```python
from build123d import *

# Parameters (mm, degrees)
CROQUIS1_R              = 2.5
SALIENTE_EXTRUIR1_DEPTH = 6
REDONDEO1_R             = 0.5
REDONDEO2_R             = 0.2
CROQUIS3_W              = 2.5
CROQUIS3_H              = 1
REDONDEO3_R             = 0.5


with BuildPart() as part:
    # Croquis1 → Saliente-Extruir1 (new body)
    with BuildSketch(Plane(origin=(0, 0, 0), x_dir=(1, 0, 0), z_dir=(0, 1, 0))):
        Polygon((-2.886751346, 5), (-5.773502692, 0), (-2.886751346, -5), (2.886751346, -5), (5.773502692, 0), (2.886751346, 5), align=None)
        Circle(CROQUIS1_R, mode=Mode.SUBTRACT)
    extrude(amount=SALIENTE_EXTRUIR1_DEPTH)

    # Redondeo1
    redondeo1_edges = [part.edges().sort_by_distance(p)[0] for p in [
        (2.886751346, 3, -5),
        (5.773502692, 3, 0),
        (2.886751346, 3, 5),
        (-2.886751346, 3, 5),
        (-5.773502692, 3, 0),
        (-2.886751346, 3, -5),
    ]]
    fillet(redondeo1_edges, radius=REDONDEO1_R)

    # Redondeo2
    redondeo2_edges = [part.edges().sort_by_distance(p)[0] for p in [
        (-4.330127019, 0, -2.5),
        (-4.330127019, 6, -2.5),
        (0, 0, -5),
        (4.330127019, 0, -2.5),
        (4.330127019, 0, 2.5),
        (0, 0, 5),
        (-4.330127019, 0, 2.5),
        (-2.848076211, 0, 4.933012702),
        (-5.696152423, 0, 0),
        (2.848076211, 0, 4.933012702),
        (5.696152423, 0, 0),
        (2.848076211, 0, -4.933012702),
        (-2.848076211, 0, -4.933012702),
        (0, 6, -5),
        (-4.330127019, 6, 2.5),
        (0, 6, 5),
        (4.330127019, 6, 2.5),
        (4.330127019, 6, -2.5),
        (-2.848076211, 6, 4.933012702),
        (-5.696152423, 6, 0),
        (2.848076211, 6, 4.933012702),
        (5.696152423, 6, 0),
        (2.848076211, 6, -4.933012702),
        (-2.848076211, 6, -4.933012702),
    ]]
    fillet(redondeo2_edges, radius=REDONDEO2_R)

    # Croquis3 → Cortar-Revolución1 (revolve, cut)
    with BuildSketch(Plane.XY):
        with Locations((-5.75, 5.5)):
            Rectangle(CROQUIS3_W, CROQUIS3_H)
    revolve(axis=Axis((0, 0, 0), (0, 1, 0)), mode=Mode.SUBTRACT)

    # Redondeo3
    redondeo3_edges = [part.edges().sort_by_distance(p)[0] for p in [
        (4.5, 6, 0),
    ]]
    fillet(redondeo3_edges, radius=REDONDEO3_R)


solid = part.part
```
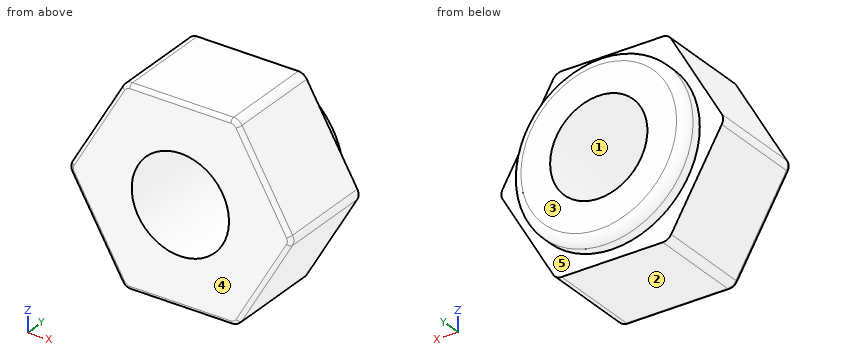
Here's how the part is built. I have some questions about the finished solid (model axes, mm). Face numbers are marked on the shaded views. A direction names the side the tool comes from. Round coordinates to 2 decimals unless told otherwise and drop trailing zeros. Order: outer loops, then holes, each group sorted by start corner. A loop starts at its lowest first (then second) coordinate and runs counter-clockwise, first axis right, second up. Notation, with made-up numbers: (68.5, 59) -> (97.5, 59) arc R8 cw to (97.5, 65) -> close; hole circle Ø10 at (20.25, -35.75). An arc over 180 degrees is marked (long way). Use a Markdown table: item, result. Add a question column.
(1) For pin 1 Ø1 at (x, y) = (-4.5, 4.5) entering from -Z; pin 2 Ø1 at (y, z) = (1, -2.5) entering from -X, each with a flat end and sliding along its axis, tell me the tip position at first contact or that it passes through.
(2) Suppose I cut it at B-B, the plane x = 0. Please give me the cut outline in (y, z), and give its area (3 significant figures).
(3) For the marked faces 4 and 5, which set-ups out of +Z, -Z, +X, -X, +Y, -Y let a thin tool reach every point of the face, with its end or its side?
(4) I need wall thicknesses on line 1 along X through (y, z) = (2.25, 0); line 2 along Z through (x, y) = (0, 4.6); line 3 along X through (y, z) = (4.05, -1). Which ranges of each line are inside material? Lowest first, please.
(5) Suppose I cut it at A-A, the plane z = 0. Please give me the cut outline in (x, y).
(6) If we mould it in two halves opening along Z, with no side actions, what happens to the marked faces 1, 2 and 3? For each: released by +Z, released by -Z, zero draft, split by the parting line, or undercut.
(7) Suppose I cut it at C-C, the plane y = 1.8. Please give me the cut outline in (x, z), and give its area (3 significant figures).
(8) Suppose I cut it at D-D, the plane y = 5.2. Please give me the cut outline in (x, z), and give its area (3 significant figures).
Verdict:
| question | item | result |
|---|---|---|
| 1 | pin 1 | z = -3.07 |
| 1 | pin 2 | x = -4.62 |
| 2 | outline | (0, -4.8) arc R0.2 ccw to (0.2, -5) -> (5, -5) -> (5, -4.5) -> (5.5, -4.5) arc R0.5 ccw to (6, -4) -> (6, -2.5) -> (0, -2.5) -> close; (0, 2.5) -> (6, 2.5) -> (6, 4) arc R0.5 ccw to (5.5, 4.5) -> (5, 4.5) -> (5, 5) -> (0.2, 5) arc R0.2 ccw to (0, 4.8) -> close |
| 2 | area | 28.9 mm2 |
| 3 | face 4 | +Z, -Z, +X, -X, -Y |
| 3 | face 5 | +Y |
| 4 | line 1 | -5.7 to -2.5, 2.5 to 5.7 |
| 4 | line 2 | -5 to -2.5, 2.5 to 5 |
| 4 | line 3 | -5.2 to -2.29, 2.29 to 5.2 |
| 5 | outline | (-5.7, 0.2) arc R0.2 ccw to (-5.5, 0) -> (-2.5, 0) -> (-2.5, 6) -> (-4, 6) arc R0.5 ccw to (-4.5, 5.5) -> (-4.5, 5) -> (-5.7, 5) -> close; (2.5, 0) -> (5.5, 0) arc R0.2 ccw to (5.7, 0.2) -> (5.7, 5) -> (4.5, 5) -> (4.5, 5.5) arc R0.5 ccw to (4, 6) -> (2.5, 6) -> close |
| 6 | face 1 | undercut |
| 6 | face 2 | released by -Z |
| 6 | face 3 | zero draft |
| 7 | outline | (-5.63, -0.25) -> (-3.03, -4.75) arc R0.5 ccw to (-2.6, -5) -> (2.6, -5) arc R0.5 ccw to (3.03, -4.75) -> (5.63, -0.25) arc R0.5 ccw to (5.63, 0.25) -> (3.03, 4.75) arc R0.5 ccw to (2.6, 5) -> (-2.6, 5) arc R0.5 ccw to (-3.03, 4.75) -> (-5.63, 0.25) arc R0.5 ccw to start; hole circle Ø5 at (0, 0) |
| 7 | area | 66.9 mm2 |
| 8 | outline | circle Ø9 at (0, 0); hole circle Ø5 at (0, 0) |
| 8 | area | 44.0 mm2 |
